Input: dimensioned drawing with shaded views. Units: mm. Origin: part minimum x, y, z. Round coordinates to 2 decimals unless told otherwise and drop trailing zeros. Loops run counter-clockwise (first coordinate to the right, second up) from the corner with the lowest first, then second, coordinate; pieces in that order, holes last. Notation, with made-up numbers: M -2.75,57 L 46.25,57 A17 cw 46.25,88 Z; hole C 15.25,-14.75 d9. An arc over 180 degrees is marked long. Answer as a JSON object with one key per item and string values.
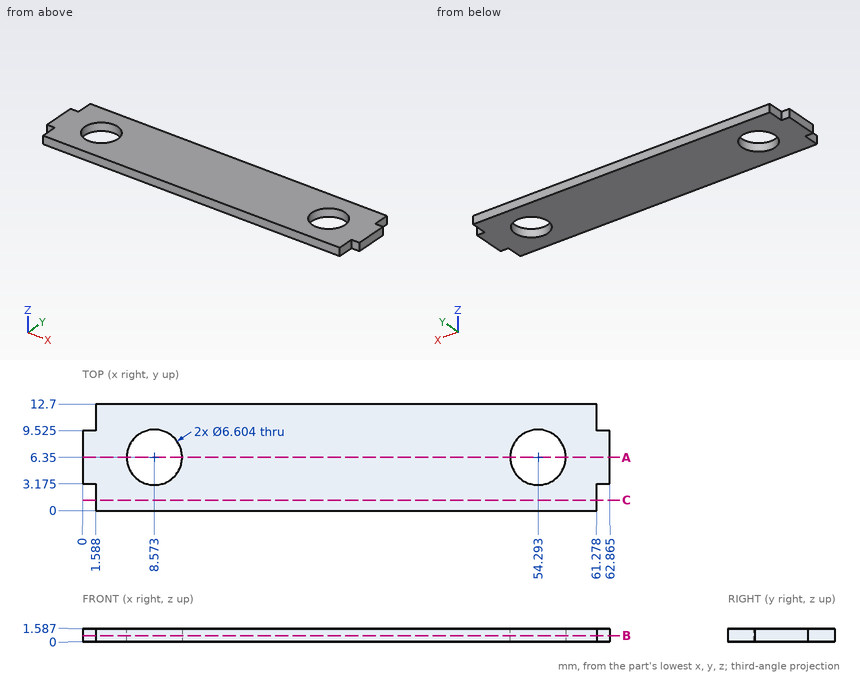
Item 1: Line query: probe 1 along X at (y, z) = (6.5, 1.5) (1 decimal); probe 2 along X at (y, z) = (7.75, 0.75) (1 decimal); probe 3 along Y at (x, z) = (10.5, 1.4). Output: solid intervals per line, ascending. Write a range as from..to.
Answer sheet:
{"probe 1": "x = 0..5.3, 11.9..51, 57.6..62.9", "probe 2": "x = 0..5.6, 11.6..51.3, 57.3..62.9", "probe 3": "y = 0..3.67, 9.03..12.7"}
Item 2: Section A-A on y = 6.35. Return the cut outline in (x, z) (1 decimal).
Answer sheet:
{"outline": "M 0,0 L 5.3,0 L 5.3,1.6 L 0,1.6 Z; M 11.9,0 L 51,0 L 51,1.6 L 11.9,1.6 Z; M 57.6,0 L 62.9,0 L 62.9,1.6 L 57.6,1.6 Z"}
Item 3: Section C-C on y = 1.25. Return the cut outline in (x, z).
Answer sheet:
{"outline": "M 1.59,0 L 61.28,0 L 61.28,1.59 L 1.59,1.59 Z"}
Item 4: Section B-B on z = 0.75. Give the number of separate pieces and of enclosed holes in the cut face, then the cut area to 3 significant figures.
Answer sheet:
{"separate pieces": "1", "enclosed holes": "2", "area": "710 mm²"}
Item 5: Contact query for flat-ended pins moving along their axis: pin 1 Ø0.5 at (x, z) = (1, 1) entering from +Y (1 decimal); pin 2 Ø0.5 at (y, z) = (1.5, 0.5) entering from -X; pin 3 Ø0.5 at (x, z) = (62, 1) entering from -Y (1 decimal). Output: stop coordinate, or through.
Answer sheet:
{"pin 1": "stops at y = 9.5", "pin 2": "stops at x = 1.59", "pin 3": "stops at y = 3.2"}
